Input: dimensioned drawing with shaded views. Units: mm. Origin: part minimum x, y, z. Round coordinates to 2 decimals unless told otherwise and drop trailing zeros. Write each loop counter-clockwise with the first axis right and the second up, starting at its lowest first coordinate (ties: lowest second). Pieces come first, ordered by that corner, then holes. Notation, with made-up numbers: (42, -6) -> (57, -6) arc R25 ccw to (57, 30) -> close; hole circle Ø8 at (23, 53). An arc over 180 degrees is marked (long way). Use one line per item in the form item = value. Start each with the question number.
1. Cut plane B-B, the plane x = 22. Return the cut outline in (y, z).
2. Cut plane C-C, the plane x = 32.25. Return the cut outline in (y, z).
3. Cut plane D-D, the plane z = 0.8. Return the cut outline in (x, y), plus the area to 3 significant figures.
4. Line query: L1, parallel to Y at x = 32.25, z = 0.55 (1 decimal); L2, parallel to Y at x = 22, z = 1; L3, parallel to Y at x = 23.5, z = 0.2. Output: solid intervals per line, ascending.
5. Cut plane A-A, the plane y = 22. Return the cut outline in (x, z).
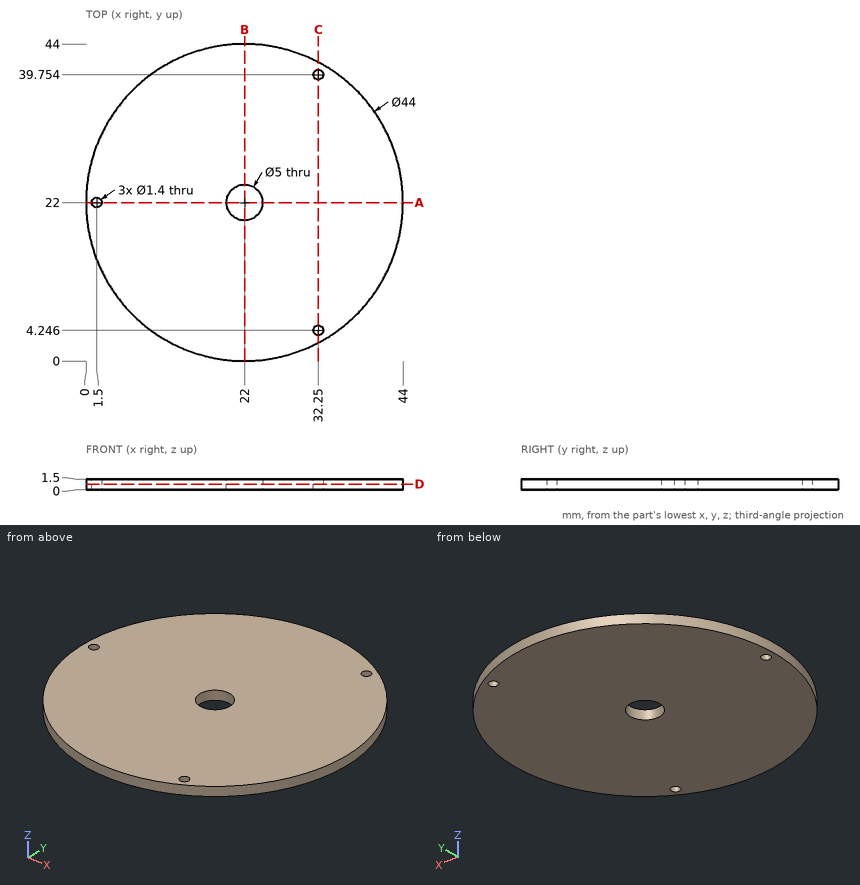
Outcome:
q1.outline = (0, 0) -> (19.5, 0) -> (19.5, 1.5) -> (0, 1.5) -> close; (24.5, 0) -> (44, 0) -> (44, 1.5) -> (24.5, 1.5) -> close
q2.outline = (2.53, 0) -> (3.55, 0) -> (3.55, 1.5) -> (2.53, 1.5) -> close; (4.95, 0) -> (39.05, 0) -> (39.05, 1.5) -> (4.95, 1.5) -> close; (40.45, 0) -> (41.47, 0) -> (41.47, 1.5) -> (40.45, 1.5) -> close
q3.outline = circle Ø44 at (22, 22); hole circle Ø1.4 at (1.5, 22); hole circle Ø5 at (22, 22); hole circle Ø1.4 at (32.25, 4.25); hole circle Ø1.4 at (32.25, 39.75)
q3.area = 1,500 mm^2
q4.L1 = 2.5 to 3.5, 4.9 to 39.1, 40.5 to 41.5
q4.L2 = 0 to 19.5, 24.5 to 44
q4.L3 = 0.05 to 20, 24 to 43.95
q5.outline = (0, 0) -> (0.8, 0) -> (0.8, 1.5) -> (0, 1.5) -> close; (2.2, 0) -> (19.5, 0) -> (19.5, 1.5) -> (2.2, 1.5) -> close; (24.5, 0) -> (44, 0) -> (44, 1.5) -> (24.5, 1.5) -> close
